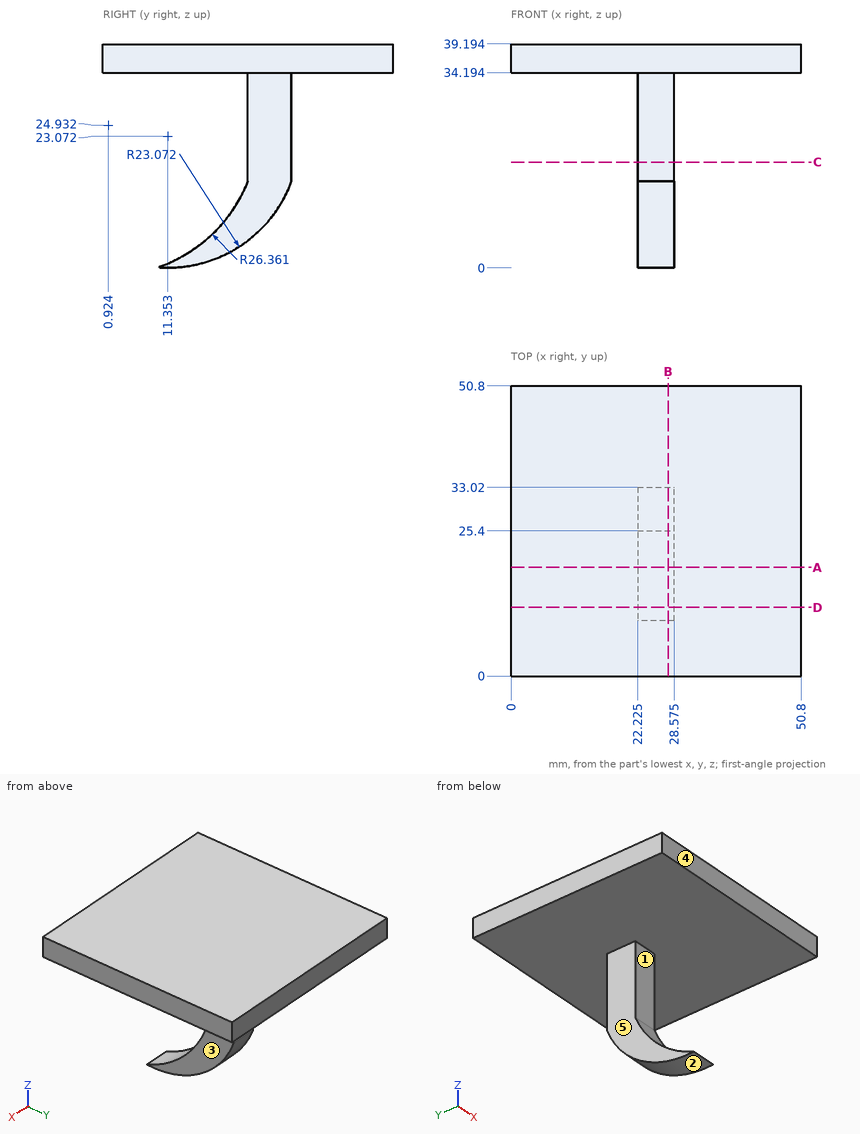
Verification items for this drawing (mm, ordinates from the low corner). A direction names the side the tool comes from. Round coordinates to 2 decimals unless told otherwise and drop trailing zeros. Order: outer loops, then holes, each group sorted by start corner. A loop starts at its lowest first (then second) coordinate and runs counter-clockwise, first axis right, second up. Notation, with made-up numbers: (25, 60) - (30, 60) arc R22 ccw to (30, 67) - close; hole circle Ø7 at (37.25, 22.5). An arc over 180 degrees is marked (long way). Use CSV: the item, a comma, the result in double quotes.
(1) Thickness scan on probe 1 along Z at (x, y) = (33, 9); probe 2 along X at (y, z) = (31, 28.5) (1 decimal); probe 3 along Y at (x, z) = (22.5, 26.5). Record the ranges inside material, lowest first. Write a range as from..to.
Entries:
probe 1,"34.19..39.19"
probe 2,"22.2..28.6"
probe 3,"25.4..33.02"
(2) Section check D-D on y = 12. Record the boundary of the cut face in (x, z) (1 decimal).
Entries:
outline,"(0, 34.2) - (50.8, 34.2) - (50.8, 39.2) - (0, 39.2) - close; (22.2, 0) - (28.6, 0) - (28.6, 1) - (22.2, 1) - close"
(3) Section check A-A on y = 19. Record the boundary of the cut face in (x, z) (1 decimal).
Entries:
outline,"(0, 34.2) - (50.8, 34.2) - (50.8, 39.2) - (0, 39.2) - close; (22.2, 1.3) - (28.6, 1.3) - (28.6, 5.7) - (22.2, 5.7) - close"
(4) Section check B-B on x = 27.5. Record the boundary of the cut face in (y, z), and give its area (3 significant figures).
Entries:
outline,"(0, 34.19) - (25.4, 34.19) - (25.4, 15.14) arc R26.36 cw to (9.66, 0.06) arc R23.07 ccw to (33.02, 15.14) - (33.02, 34.19) - (50.8, 34.19) - (50.8, 39.19) - (0, 39.19) - close"
area,"510 mm^2"
(5) Access from +Z, -Z, +X, -X, +Y, -Y to the whole of each face (thin tool, end or side, straight path). Record for the marked faces 4 and 5.
Entries:
face 4,"+Z, -Z, +X, -X, -Y"
face 5,"-Z, -X, +Y, -Y"
(6) Section check C-C on z = 18.5. Record the boundary of the cut face in (x, y) (1 decimal), and give its area (3 significant figures).
Entries:
outline,"(22.2, 25.4) - (28.6, 25.4) - (28.6, 33) - (22.2, 33) - close"
area,"48.4 mm^2"
(7) Gauge pin test, flat ends, axial feed: pin 1 Ø6 at (x, z) = (25.5, 29) entering from -Y; pin 2 Ø5 at (x, z) = (26.5, 24) entering from +Y; pin 3 Ø12 at (y, z) = (42, 22.5) entering from +X; pin 4 Ø7 at (y, z) = (26.5, 25) entering from +X (3 decimals). Record the tip position at first contact, or that the pin passes through.
Entries:
pin 1,"y = 25.4"
pin 2,"y = 33.02"
pin 3,"through"
pin 4,"x = 28.575"
(8) Mould release check, pull along Z, two halves, no side actions. Record for the marked faces 1, 2 and 3: released by +Z, released by -Z, zero draft, split by the parting line, or undercut.
Entries:
face 1,"undercut"
face 2,"released by -Z"
face 3,"zero draft"
